CAD build for the part. Positions are in the model's coordinates, mm. Face numbers are marked on the shaded views. A direction names the side the tool comes from. Give positions to 0.01 mm unless a question says otherwise; leave off trailing zeros. Write each loop counter-clockwise with the first axis right and the second up, starting at its lowest first coordinate (ties: lowest second). Pieces come first, ordered by that corner, then holes. Notation, with made-up numbers: (85.25, -18) -> (144.25, -18) arc R24 ccw to (144.25, 19) -> close; hole circle Ø1 at (-6.5, 34.25). An arc over 180 degrees is marked (long way). Answer as a JSON object with one key per item and string values.
```python
from build123d import *

# Parameters (mm, degrees)
BOSS_EXTRUDE1_DEPTH = 50
SKETCH21_W          = 50
SKETCH21_H          = 3
TAPPED_HOLE4_D      = 3.3
TAPPED_HOLE4_DEPTH  = 11.5
TAPPED_HOLE4_TIP    = 0.991420021
TAPPED_HOLE5_D      = 3.3
TAPPED_HOLE5_DEPTH  = 11.5
TAPPED_HOLE5_TIP    = 0.991420021


with BuildPart() as part:
    # Sketch1 → Boss-Extrude1 (new body)
    with BuildSketch(Plane(origin=(0, 0, 0), x_dir=(0, 0, -1), z_dir=(1, 0, 0))):
        Polygon((0, -3.464101615), (3, -1.732050808), (3, 1.732050808), (0, 3.464101615), (-3, 1.732050808), (-3, -1.732050808), align=None)
    extrude(amount=BOSS_EXTRUDE1_DEPTH)

    # Sketch2 → Cut-Revolve1 (revolve, cut)
    with BuildSketch(Plane.XY):
        Polygon((0, 3.464101615), (0.267949192, 3.464101615), (0, 3), align=None)
        Polygon((49.732050808, 3.464101615), (50, 3), (50, 3.464101615), align=None)
    revolve(axis=Axis((0, 0, 0), (1, 0, 0)), mode=Mode.SUBTRACT)

    # Sketch21 → Revolve1 (revolve)
    with BuildSketch(Plane.XY):
        with Locations((25, 1.5)):
            Rectangle(SKETCH21_W, SKETCH21_H)
    revolve(axis=Axis((0, 0, 0), (1, 0, 0)))

    # Tapped Hole4
    with Locations(Plane(origin=(0, -0.118657881, 0.00506752), x_dir=(0, 0, -1), z_dir=(-1, 0, 0))):
        with Locations((0.00506752, -0.118657881)):
            Hole(TAPPED_HOLE4_D / 2, depth=TAPPED_HOLE4_DEPTH)
            with Locations((0, 0, -(TAPPED_HOLE4_DEPTH + TAPPED_HOLE4_TIP / 2))):  # 118° drill point
                Cone(0, TAPPED_HOLE4_D / 2, TAPPED_HOLE4_TIP, mode=Mode.SUBTRACT)

    # Tapped Hole5
    with Locations(Plane(origin=(50, 0.843813549, 0.0751412), x_dir=(0, 0, -1), z_dir=(1, 0, 0))):
        with Locations((0.0751412, -0.843813549)):
            Hole(TAPPED_HOLE5_D / 2, depth=TAPPED_HOLE5_DEPTH)
            with Locations((0, 0, -(TAPPED_HOLE5_DEPTH + TAPPED_HOLE5_TIP / 2))):  # 118° drill point
                Cone(0, TAPPED_HOLE5_D / 2, TAPPED_HOLE5_TIP, mode=Mode.SUBTRACT)


solid = part.part
```
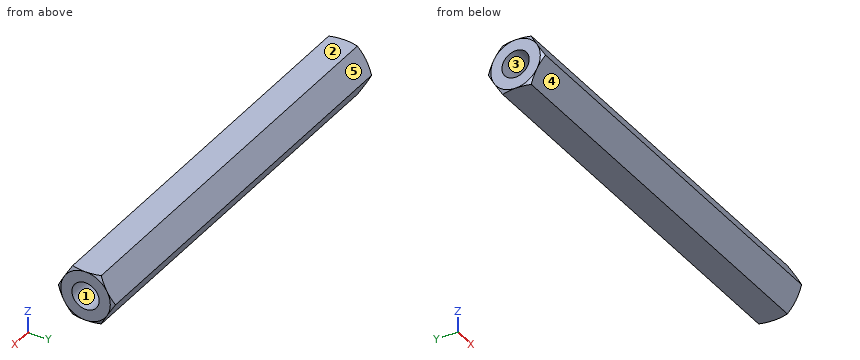
1) Pin check, flat tip, straight feed: pin 1 (3 mm diameter, centred on x = 29, z = -0.5, fed in from +Y). Stop position of the tip, or through.
Model answer:
{"pin 1": "stops at y = 3.46"}
2) Slice it at B-B (x = 36). List the corners of the cut face in (y, z).
Model answer:
{"outline": "(-3.46, 0) -> (-1.73, -3) -> (1.73, -3) -> (3.46, 0) -> (1.73, 3) -> (-1.73, 3) -> close"}
3) Slice it at A-A (x = 8.5). List the corners of the cut face in (y, z).
Model answer:
{"outline": "(-3.46, 0) -> (-1.73, -3) -> (1.73, -3) -> (3.46, 0) -> (1.73, 3) -> (-1.73, 3) -> close; hole circle Ø3.3 at (0, 0)"}
4) Wall check: probe 1 along Y at (x, z) = (43, 0); probe 2 along Z at (x, y) = (41.25, 0); probe 3 along Z at (x, y) = (42, 1). Give the ranges that are in metal, low to high.
Model answer:
{"probe 1": "y = -3.46 to -1.65, 1.65 to 3.46", "probe 2": "z = -3 to -1.65, 1.65 to 3", "probe 3": "z = -3 to -1.31, 1.31 to 3"}
5) Mould opens along Z. For the marked faces 3, 4 and 5 say: released by +Z, released by -Z, zero draft, split by the parting line, or undercut.
Model answer:
{"face 3": "undercut", "face 4": "released by -Z", "face 5": "released by +Z"}
6) 3-axis set-ups, long thin cutter, end or side, ignore diameter. For the marked faces 1 and 2: which of +Z, -Z, +X, -X, +Y, -Y reach the whole face in a straight line?
Model answer:
{"face 1": "+X", "face 2": "+Z, +X, -X, +Y, -Y"}
